Check sheet for the drawn part. Datum: minimum x, y, z corner. Units: mm. A direction names the side the tool comes from. Give positions to 0.01 mm unless a question says otherwise; leave off trailing zeros. Write each loop counter-clockwise with the first axis right and the second up, starting at its lowest first coordinate (ties: lowest second). Pieces come first, ordered by that corner, then holes. Notation, with made-up numbers: M 40,82 L 69,82 A11 cw 69,87 Z; hole C -30.75,35 d8. An arc over 180 degrees is marked long. Write item = value, one per line. Start each with the question number.
1) Scan lines: L1, parallel to Y at x = 12.5, z = 26.5; L2, parallel to X at y = 27, z = 14. Record each from-to range of solid material in increasing order.
2) Sectioned sample at D-D, the plane y = 29. Record the cut outline in (x, z).
3) Gauge pin test, flat ends, axial feed: pin 1 (6.5 mm diameter, centred on x = 4.5, y = 20.5, fed in from +Z); pin 2 (1 mm diameter, centred on x = 16, y = 30, fed in from +Z). Record the tip position at first contact, or that the pin passes through.
4) Draft check along Y on the marked faces 1, 2, 3 and 4. Enter one of: pulls with the +Y half, pulls with the -Y half, needs draft (parallel to the pull), parting line crosses it, or undercut.
5) Sectioned sample at B-B, the plane y = 19. Record the cut outline in (x, z).
6) Sectioned sample at C-C, the plane x = 11.25. Record the cut outline in (y, z), then the cut area to 3 significant figures.
7) Sectioned sample at A-A, the plane z = 30. Record the cut outline in (x, y).
8) Set-up check for the marked faces 5 and 6: record each of +Z, -Z, +X, -X, +Y, -Y from which the full face is reachable in a straight line by a thin tool's end or side.
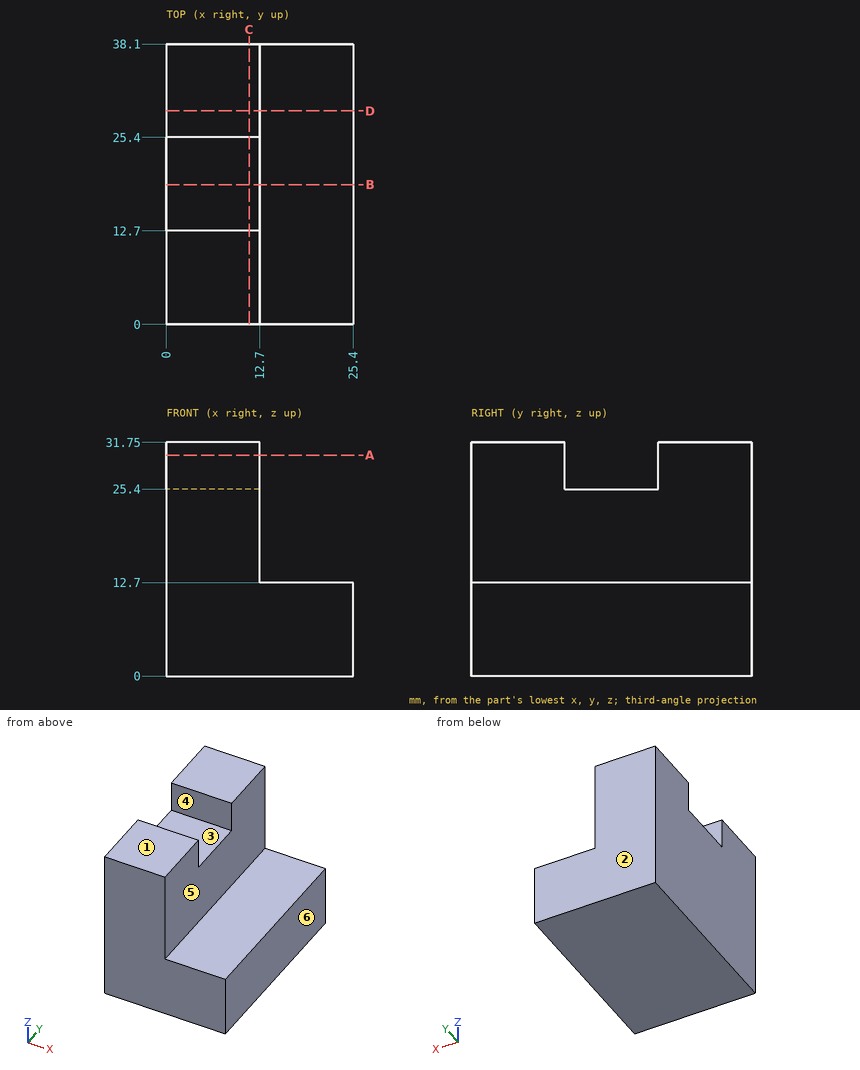
Data:
q1.L1 = 0 to 12.7, 25.4 to 38.1
q1.L2 = 0 to 12.7
q2.outline = M 0,0 L 25.4,0 L 25.4,12.7 L 12.7,12.7 L 12.7,31.75 L 0,31.75 Z
q3.pin_1 = 25.4
q3.pin_2 = 12.7
q4.face_1 = needs draft
q4.face_2 = pulls with the +Y half
q4.face_3 = undercut
q4.face_4 = undercut
q5.outline = M 0,0 L 25.4,0 L 25.4,12.7 L 12.7,12.7 L 12.7,25.4 L 0,25.4 Z
q6.outline = M 0,0 L 38.1,0 L 38.1,31.75 L 25.4,31.75 L 25.4,25.4 L 12.7,25.4 L 12.7,31.75 L 0,31.75 Z
q6.area = 1,130 mm2
q7.outline = M 0,0 L 12.7,0 L 12.7,12.7 L 0,12.7 Z; M 0,25.4 L 12.7,25.4 L 12.7,38.1 L 0,38.1 Z
q8.face_5 = +Z, +X, +Y, -Y
q8.face_6 = +Z, -Z, +X, +Y, -Y
